Geometry check sheet. Reference: the model listing, model coordinates, mm. Face numbers are marked on the shaded views. A direction names the side the tool comes from. Give positions to 0.01 mm unless a question says otherwise; leave off trailing zeros. Order: outer loops, then holes, each group sorted by start corner. A loop starts at its lowest first (then second) coordinate and runs counter-clockwise, first axis right, second up. Notation, with made-up numbers: M 76.5,41 L 132.5,41 A38 ccw 132.5,79 Z; hole C -4,15 d3. An arc over 180 degrees is marked long. Answer as CSV lines item,"result".
from build123d import *

# Parameters (mm, degrees)
F1_DEPTH = 6.5


# Not quite as in the source:
# - a feature names something its author has since deleted; it is built from what else it names


with BuildPart() as f1:
    # F0 (on Top) → F1 (new body)
    with BuildSketch(Plane.XY):
        with BuildLine():
            Line((10, 13.9658923334), (10, 5.6794919243))
            Line((10, 5.6794919243), (10.6173677664, 4.610179586))
            Line((10.6173677664, 4.610179586), (17.4592921435, 1.0460193523))
            ThreePointArc((17.4592921435, 1.0460193523), (12.2366972109, 6.6440014162), (10, 13.9658923334))
        make_face()
        with BuildLine():
            Line((5, 14.3397459622), (10, 5.6794919243))
            Line((10, 5.6794919243), (10, 13.9658923334))
            Line((10, 13.9658923334), (10, 23))
            ThreePointArc((10, 23), (8.6602540378, 18), (5, 14.3397459622))
        make_face()
        with BuildLine():
            Line((17.4592921435, 1.0460193523), (10.6173677664, 4.610179586))
            Line((10.6173677664, 4.610179586), (14.918584287, -2.8397459622))
            ThreePointArc((14.918584287, -2.8397459622), (19.4852389907, -1.5093938195), (24.1499344795, -2.4393336035))
            Line((24.1499344795, -2.4393336035), (17.4592921435, 1.0460193523))
        make_face()
        with BuildLine():
            Line((-7.4592921435, -15.6551270189), (-0.5795069127, -11.5))
            Line((-0.5795069127, -11.5), (-9.918584287, -11.5))
            ThreePointArc((-9.918584287, -11.5), (-11.1613785992, -16.328182737), (-14.5808539954, -19.9562778652))
            Line((-14.5808539954, -19.9562778652), (-7.4592921435, -15.6551270189))
        make_face()
        with BuildLine():
            Line((0.5795069127, -11.5), (-0.5795069127, -11.5))
            Line((-0.5795069127, -11.5), (-7.4592921435, -15.6551270189))
            ThreePointArc((-7.4592921435, -15.6551270189), (0, -13.9312181655), (7.4592921435, -15.6551270189))
            Line((7.4592921435, -15.6551270189), (0.5795069127, -11.5))
        make_face()
        with BuildLine():
            Line((9.918584287, -11.5), (0.5795069127, -11.5))
            Line((0.5795069127, -11.5), (7.4592921435, -15.6551270189))
            Line((7.4592921435, -15.6551270189), (14.5808539954, -19.9562778652))
            ThreePointArc((14.5808539954, -19.9562778652), (11.1613785992, -16.328182737), (9.918584287, -11.5))
        make_face()
        with BuildLine():
            Line((0, 23), (5, 14.3397459622))
            ThreePointArc((5, 14.3397459622), (8.6602540378, 18), (10, 23))
            Line((10, 23), (0, 23))
        make_face()
        with BuildLine():
            ThreePointArc((24.1499344795, -2.4393336035), (19.4852389907, -1.5093938195), (14.918584287, -2.8397459622))
            Line((14.918584287, -2.8397459622), (19.918584287, -11.5))
            Line((19.918584287, -11.5), (24.918584287, -2.8397459622))
            Line((24.918584287, -2.8397459622), (24.1499344795, -2.4393336035))
        make_face()
        with BuildLine():
            Line((-10, 13.9658923334), (-10, 5.6794919243))
            Line((-10, 5.6794919243), (-5, 14.3397459622))
            ThreePointArc((-5, 14.3397459622), (-8.6602540378, 18), (-10, 23))
            Line((-10, 23), (-10, 13.9658923334))
        make_face()
        with BuildLine():
            Line((-10.6173677664, 4.610179586), (-10, 5.6794919243))
            Line((-10, 5.6794919243), (-10, 13.9658923334))
            ThreePointArc((-10, 13.9658923334), (-12.2366972109, 6.6440014162), (-17.4592921435, 1.0460193523))
            Line((-17.4592921435, 1.0460193523), (-10.6173677664, 4.610179586))
        make_face()
        with BuildLine():
            Line((-14.918584287, -2.8397459622), (-10.6173677664, 4.610179586))
            Line((-10.6173677664, 4.610179586), (-17.4592921435, 1.0460193523))
            Line((-17.4592921435, 1.0460193523), (-24.1499344795, -2.4393336035))
            ThreePointArc((-24.1499344795, -2.4393336035), (-19.4852389907, -1.5093938195), (-14.918584287, -2.8397459622))
        make_face()
        with BuildLine():
            ThreePointArc((-14.5808539954, -19.9562778652), (-11.1613785992, -16.328182737), (-9.918584287, -11.5))
            Line((-9.918584287, -11.5), (-19.918584287, -11.5))
            Line((-19.918584287, -11.5), (-14.918584287, -20.1602540378))
            Line((-14.918584287, -20.1602540378), (-14.5808539954, -19.9562778652))
        make_face()
        with BuildLine():
            Line((19.918584287, -11.5), (9.918584287, -11.5))
            ThreePointArc((9.918584287, -11.5), (11.1613785992, -16.328182737), (14.5808539954, -19.9562778652))
            Line((14.5808539954, -19.9562778652), (14.918584287, -20.1602540378))
            Line((14.918584287, -20.1602540378), (19.918584287, -11.5))
        make_face()
        with BuildLine():
            Line((-5, 14.3397459622), (0, 23))
            Line((0, 23), (-10, 23))
            ThreePointArc((-10, 23), (-8.6602540378, 18), (-5, 14.3397459622))
        make_face()
        with BuildLine():
            Line((-10, 23), (0, 23))
            Line((0, 23), (10, 23))
            ThreePointArc((10, 23), (0, 33), (-10, 23))
        make_face()
        with BuildLine():
            Line((24.918584287, -2.8397459622), (19.918584287, -11.5))
            Line((19.918584287, -11.5), (14.918584287, -20.1602540378))
            ThreePointArc((14.918584287, -20.1602540378), (24.918584287, -20.1602540378), (29.918584287, -11.5))
            ThreePointArc((29.918584287, -11.5), (28.5788383249, -6.5), (24.918584287, -2.8397459622))
        make_face()
        with BuildLine():
            ThreePointArc((24.918584287, -2.8397459622), (24.538599342, -2.6312086003), (24.1499344795, -2.4393336035))
            Line((24.1499344795, -2.4393336035), (24.918584287, -2.8397459622))
        make_face()
        with BuildLine():
            Line((-19.918584287, -11.5), (-14.918584287, -2.8397459622))
            ThreePointArc((-14.918584287, -2.8397459622), (-19.4852389907, -1.5093938195), (-24.1499344795, -2.4393336035))
            Line((-24.1499344795, -2.4393336035), (-24.918584287, -2.8397459622))
            Line((-24.918584287, -2.8397459622), (-19.918584287, -11.5))
        make_face()
        with BuildLine():
            Line((-14.918584287, -20.1602540378), (-19.918584287, -11.5))
            Line((-19.918584287, -11.5), (-24.918584287, -2.8397459622))
            ThreePointArc((-24.918584287, -2.8397459622), (-28.5788383249, -16.5), (-14.918584287, -20.1602540378))
        make_face()
        with BuildLine():
            ThreePointArc((-14.918584287, -20.1602540378), (-14.7487130637, -20.0599317482), (-14.5808539954, -19.9562778652))
            Line((-14.5808539954, -19.9562778652), (-14.918584287, -20.1602540378))
        make_face()
        with BuildLine():
            Line((14.918584287, -20.1602540378), (14.5808539954, -19.9562778652))
            ThreePointArc((14.5808539954, -19.9562778652), (14.7487130637, -20.0599317482), (14.918584287, -20.1602540378))
        make_face()
        with BuildLine():
            Line((-24.918584287, -2.8397459622), (-24.1499344795, -2.4393336035))
            ThreePointArc((-24.1499344795, -2.4393336035), (-24.538599342, -2.6312086003), (-24.918584287, -2.8397459622))
        make_face()
        with BuildLine():
            Line((-0.5795069127, -11.5), (0, -11.15))
            ThreePointArc((0, -11.15), (-9.468682565, -5.8878307111), (-10, 4.9317846668))
            Line((-10, 4.9317846668), (-10.6173677664, 4.610179586))
            Line((-10.6173677664, 4.610179586), (-14.918584287, -2.8397459622))
            ThreePointArc((-14.918584287, -2.8397459622), (-11.2583302492, -6.5), (-9.918584287, -11.5))
            Line((-9.918584287, -11.5), (-0.5795069127, -11.5))
        make_face()
        with BuildLine():
            Line((-19.918584287, -11.5), (-9.918584287, -11.5))
            ThreePointArc((-9.918584287, -11.5), (-11.2583302492, -6.5), (-14.918584287, -2.8397459622))
            Line((-14.918584287, -2.8397459622), (-19.918584287, -11.5))
        make_face()
        Polygon((-10.6173677664, 4.610179586), (-10, 4.9317846668), (-10, 5.6794919243), align=None)
        with BuildLine():
            ThreePointArc((-10, 4.9317846668), (-5.8878307111, 9.468682565), (0, 11.15))
            Line((0, 11.15), (0, 13))
            ThreePointArc((0, 13), (-2.588190451, 13.3407417371), (-5, 14.3397459622))
            Line((-5, 14.3397459622), (-10, 5.6794919243))
            Line((-10, 5.6794919243), (-10, 4.9317846668))
        make_face()
        with BuildLine():
            ThreePointArc((-5, 14.3397459622), (-2.588190451, 13.3407417371), (0, 13))
            Line((0, 13), (0, 23))
            Line((0, 23), (-5, 14.3397459622))
        make_face()
        with BuildLine():
            Line((0, 23), (0, 13))
            ThreePointArc((0, 13), (2.588190451, 13.3407417371), (5, 14.3397459622))
            Line((5, 14.3397459622), (0, 23))
        make_face()
        with BuildLine():
            ThreePointArc((0, 11.15), (5.8878307111, 9.468682565), (10, 4.9317846668))
            Line((10, 4.9317846668), (10, 5.6794919243))
            Line((10, 5.6794919243), (5, 14.3397459622))
            ThreePointArc((5, 14.3397459622), (2.588190451, 13.3407417371), (0, 13))
            Line((0, 13), (0, 11.15))
        make_face()
        Polygon((10, 5.6794919243), (10, 4.9317846668), (10.6173677664, 4.610179586), align=None)
        with BuildLine():
            ThreePointArc((10, 4.9317846668), (10.8586946729, 2.5320446284), (11.15, 0))
            ThreePointArc((11.15, 0), (7.8842406102, -7.8842406102), (0, -11.15))
            Line((0, -11.15), (0.5795069127, -11.5))
            Line((0.5795069127, -11.5), (9.918584287, -11.5))
            ThreePointArc((9.918584287, -11.5), (11.2583302492, -6.5), (14.918584287, -2.8397459622))
            Line((14.918584287, -2.8397459622), (10.6173677664, 4.610179586))
            Line((10.6173677664, 4.610179586), (10, 4.9317846668))
        make_face()
        with BuildLine():
            Line((19.918584287, -11.5), (14.918584287, -2.8397459622))
            ThreePointArc((14.918584287, -2.8397459622), (11.2583302492, -6.5), (9.918584287, -11.5))
            Line((9.918584287, -11.5), (19.918584287, -11.5))
        make_face()
        Polygon((0.5795069127, -11.5), (0, -11.15), (-0.5795069127, -11.5), align=None)
    extrude(amount=F1_DEPTH)


solid = f1.part
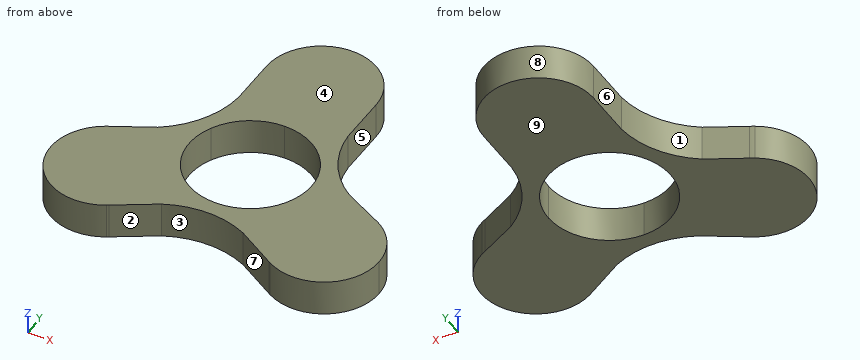
(1) Section check D-D on y = 24.5. Enter the section's corners in (x, z), then the cut area to 3 significant figures.
The answers:
outline,"M -9.89,0 L 9.89,0 L 9.89,6.5 L -9.89,6.5 Z"
area,"129 mm2"
(2) Section check C-C on x = -3. Enter the section's corners in (y, z), then the cut area to 3 significant figures.
The answers:
outline,"M -14.2,0 L -10.74,0 L -10.74,6.5 L -14.2,6.5 Z; M 10.74,0 L 32.54,0 L 32.54,6.5 L 10.74,6.5 Z"
area,"164 mm2"
(3) Gauge pin test, flat ends, axial feed: P1, Ø1.5, axis at y = 18.5, z = 5, coming from the +X side; P2, Ø3, axis at y = 17.5, z = 4, coming from the -X side; P3, Ø3, axis at y = 8.5, z = 2, coming from the -X side. Record the tip position at first contact, or that the pin passes through.
The answers:
P1,"stops at x = 10"
P2,"stops at x = -10"
P3,"stops at x = -12.04"
(4) Draft check along X on the marked faces 1, 2, 3 and 4. Enter one of: +X half, -X half, draft (parallel to the pull), parting line (faces both ways), or undercut.
The answers:
face 1,"-X half"
face 2,"undercut"
face 3,"undercut"
face 4,"draft"
(5) Section check A-A on z = 2.75. Enter the section's corners in (x, y).
The answers:
outline,"M -24.15,-2.44 A10 ccw long -14.58,-19.96 L -7.46,-15.66 A17 cw 7.46,-15.66 L 14.58,-19.96 A10 ccw long 24.15,-2.44 L 17.46,1.05 A17 cw 10,13.97 L 10,23 A10 ccw -10,23 L -10,13.97 A17 cw -17.46,1.05 Z; hole C 0,0 d22.3"
(6) Tool access check on the marked faces 5, 6, 7, 8 and 9. Record the directions out of +Z, -Z, +X, -X, +Y, -Y that give a thin tool (end or side, any length) a straight path to the whole face; none if there is none.
The answers:
face 5,"+Z, -Z, +X, +Y"
face 6,"+Z, -Z, -X, +Y"
face 7,"+Z, -Z, -Y"
face 8,"+Z, -Z, +Y"
face 9,"-Z, +X, -X, +Y, -Y"
(7) Section check B-B on y = -4.5. Enter the section's corners in (x, z).
The answers:
outline,"M -27.06,0 L -10.2,0 L -10.2,6.5 L -27.06,6.5 Z; M 10.2,0 L 27.06,0 L 27.06,6.5 L 10.2,6.5 Z"
(8) Material ranges on line 1 (X direction, y = -9, z = 6); line 2 (X direction, y = 10, z = 1); line 3 (X direction, y = 23, z = 1.5), recorded low to high.
The answers:
line 1,"x = -29.6 to -6.58, 6.58 to 29.6"
line 2,"x = -10.76 to -4.93, 4.93 to 10.76"
line 3,"x = -10 to 10"
